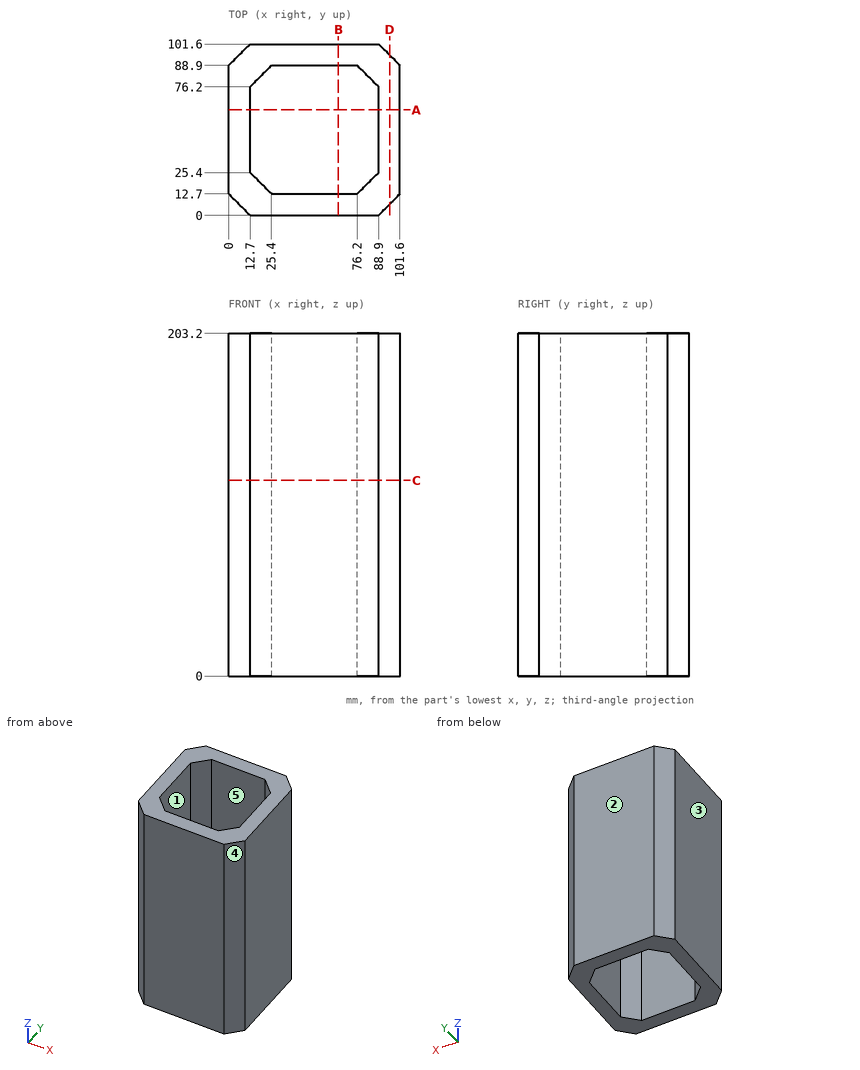
Here's the drawing with two shaded views (mm, measured from the low corner). I have some questions. A direction names the side the tool comes from. Give positions to 0.01 mm unless a question says otherwise; leave off trailing zeros. Loops run counter-clockwise (first coordinate to the right, second up) from the corner with the lowest first, then second, coordinate; pieces in that order, holes last. Notation, with made-up numbers: M -39.75,-3 L -1.75,-3 A24 ccw -1.75,31 Z; hole C 15.5,-9.75 d3. An arc over 180 degrees is marked long. Answer in a Markdown table with one row per item.
1. Suppose I cut it at D-D on x = 95.5. Write out the boundary of the cut face in (y, z).
Taken from the geometry:
| item | result |
|---|---|
| outline | M 6.6,0 L 95,0 L 95,203.2 L 6.6,203.2 Z |
2. If I drill on line 1 along Y through (x, z) = (33, 159); line 2 along Y through (x, z) = (87, 137), over which ranges is the centre line in solid material (lowest first)?
Taken from the geometry:
| item | result |
|---|---|
| line 1 | y = 0 to 12.7, 88.9 to 101.6 |
| line 2 | y = 0 to 23.5, 78.1 to 101.6 |
3. For pin 1 Ø1 at (y, z) = (11, 133.5) entering from -X, with a flat end and sliding along its axis, tell me the tip position at first contact or that it passes through.
Taken from the geometry:
| item | result |
|---|---|
| pin 1 | stops at x = 1.2 |
4. Suppose I cut it at A-A on y = 62.5. Write out the boundary of the cut face in (x, z).
Taken from the geometry:
| item | result |
|---|---|
| outline | M 0,0 L 12.7,0 L 12.7,203.2 L 0,203.2 Z; M 88.9,0 L 101.6,0 L 101.6,203.2 L 88.9,203.2 Z |
5. Which directions (+Z, -Z, +X, -X, +Y, -Y) give clear straight access to the entire face, cutting with the end or side of a thin tool? Please do the marked faces 1 and 2.
Taken from the geometry:
| item | result |
|---|---|
| face 1 | +Z, -Z |
| face 2 | +Z, -Z, +X, -X, +Y |
6. Thinking about a two-plate mould opening in Y: for the marked faces 3, 4 and 5, which applies, released by +Y, released by -Y, zero draft, split by the parting line, or undercut?
Taken from the geometry:
| item | result |
|---|---|
| face 3 | zero draft |
| face 4 | released by -Y |
| face 5 | undercut |
7. Suppose I cut it at C-C on z = 116. Write out the boundary of the cut face in (x, y), plus the area to 3 significant figures.
Taken from the geometry:
| item | result |
|---|---|
| outline | M 0,12.7 L 12.7,0 L 88.9,0 L 101.6,12.7 L 101.6,88.9 L 88.9,101.6 L 12.7,101.6 L 0,88.9 Z; hole M 12.7,25.4 L 25.4,12.7 L 76.2,12.7 L 88.9,25.4 L 88.9,76.2 L 76.2,88.9 L 25.4,88.9 L 12.7,76.2 Z |
| area | 4,520 mm² |
